Geometry check sheet. Reference: drawing and pictorial views, mm from the part's lowest x, y, z. A direction names the side the tool comes from. Round coordinates to 2 decimals unless told otherwise and drop trailing zeros. Loops run counter-clockwise (first coordinate to the right, second up) from the corner with the lowest first, then second, coordinate; pieces in that order, holes last. Notation, with made-up numbers: (-30, -13) -> (-26, -13) arc R18 cw to (-26, 9) -> close; hole circle Ø2 at (50, -34). An arc over 180 degrees is marked (long way). Use one line per item in the form item = value. Start each with the question number.
(1) Sectioned sample at D-D (y = 49). Record the cut outline in (x, z), and give its area (3 significant figures).
(2) Draft check along Y on the marked faces 3, 4 and 5. Enter one of: released by +Y, released by -Y, zero draft, split by the parting line, or undercut.
(3) Sectioned sample at A-A (y = 31.75). Record the cut outline in (x, z), and give its area (3 significant figures).
(4) Sectioned sample at B-B (x = 63.5). Record the cut outline in (y, z).
(5) Go/stop test with flat-tipped pins: pin 1 (2 mm diameter, centred on x = 61.5, z = 26, fed in from -Y); pin 2 (12 mm diameter, centred on x = 56, z = 6, fed in from +Y); pin 3 (10 mm diameter, centred on x = 63.5, y = 31.75, fed in from -Z); pin 4 (5 mm diameter, centred on x = 33.5, y = 23, fed in from +Z). Record where each tip stops, or that it passes through.
(6) Set-up check for the marked faces 1 and 2: record each of +Z, -Z, +X, -X, +Y, -Y from which the full face is reachable in a straight line by a thin tool's end or side.
(7) Sectioned sample at C-C (x = 38.1). Record the cut outline in (y, z).
(8) Material ranges on probe 1 along Y at (x, z) = (63.5, 13); probe 2 along X at (y, z) = (31, 18); probe 3 along Y at (x, z) = (73, 24), recorded low to high. Write a range as [from, to].
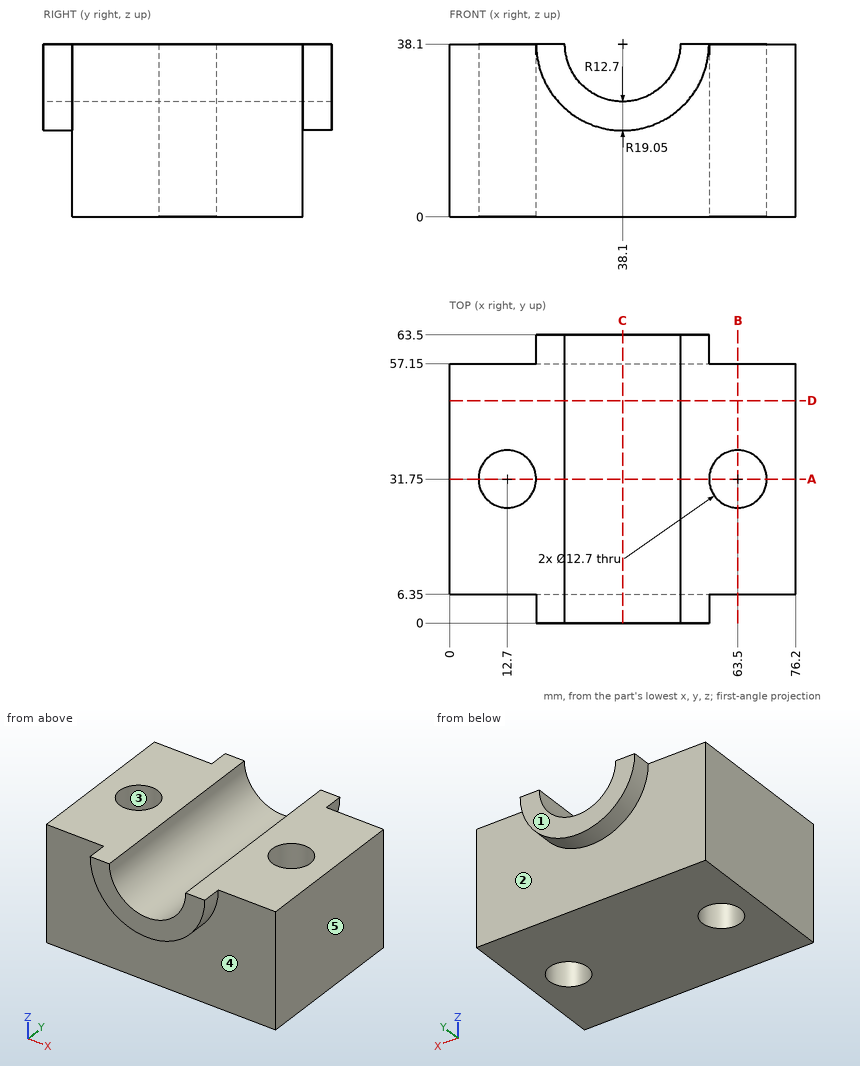
Checks:
q1.outline = (0, 0) -> (76.2, 0) -> (76.2, 38.1) -> (50.8, 38.1) arc R12.7 cw to (25.4, 38.1) -> (0, 38.1) -> close
q1.area = 2,650 mm2
q2.face_3 = undercut
q2.face_4 = released by -Y
q2.face_5 = zero draft
q3.outline = (0, 0) -> (6.35, 0) -> (6.35, 38.1) -> (0, 38.1) -> close; (19.05, 0) -> (57.15, 0) -> (57.15, 38.1) -> (50.8, 38.1) arc R12.7 cw to (25.4, 38.1) -> (19.05, 38.1) -> close; (69.85, 0) -> (76.2, 0) -> (76.2, 38.1) -> (69.85, 38.1) -> close
q3.area = 1,680 mm2
q4.outline = (6.35, 0) -> (25.4, 0) -> (25.4, 38.1) -> (6.35, 38.1) -> close; (38.1, 0) -> (57.15, 0) -> (57.15, 38.1) -> (38.1, 38.1) -> close
q5.pin_1 = 6.35
q5.pin_2 = 57.15
q5.pin_3 = through
q5.pin_4 = 27.57
q6.face_1 = +Z, -Z, +X, -X, +Y
q6.face_2 = -Z, +Y
q7.outline = (0, 19.05) -> (6.35, 19.05) -> (6.35, 0) -> (57.15, 0) -> (57.15, 19.05) -> (63.5, 19.05) -> (63.5, 25.4) -> (0, 25.4) -> close
q8.probe_1 = [6.35, 25.4], [38.1, 57.15]
q8.probe_2 = [0, 6.39], [19.01, 57.19], [69.81, 76.2]
q8.probe_3 = [6.35, 57.15]
